Design review of the part built by this model. Coordinates are the model's own, in mm. Face numbers are marked on the shaded views. A direction names the side the tool comes from. Coordinates: 2 decimals unless noted, no trailing zeros. Loops run counter-clockwise (first coordinate to the right, second up) from the corner with the lowest first, then second, coordinate; pieces in that order, holes last. Notation, with made-up numbers: M 53,23 L 71,23 A18 ccw 71,40 Z; hole C 17.5,2.5 d2. An arc over 180 degrees is marked long. Answer as a JSON object with one key per item and string values. Group by question number.
1. Machinability: for the marked faces 1 and 2, which of the approach directions +Z, -Z, +X, -X, +Y, -Y give a long, thin tool a straight path to every point of the face, cutting with its end or side? Answer none if there is none.
2. Consider section C-C (x = 14). State the section outline as (y, z) points, then the cut area to 3 significant figures.
3. Consider section A-A (x = 0). State the section outline as (y, z) points, then the cut area to 3 significant figures.
4. To check wall thickness, follow probe 1 along Y at (x, z) = (0, 0.8); probe 2 along Y at (x, z) = (0, 3.5); probe 3 along Z at (x, y) = (4, -15). State the ranges of each line that lie inside material, in increasing order.
5. Insertion check: pin 1 (1 mm diameter, centred on x = 12, z = 1.5, fed in from +Y); pin 2 (4 mm diameter, centred on x = 14, y = 0, fed in from +Z); pin 3 (4 mm diameter, centred on y = -7, z = 1, fed in from +X). Each pin has a flat end and moves straight along its axis. Give the tip position at first contact, or say it passes through.
6. Consider section D-D (z = 1). State the section outline as (x, y) points, then the cut area to 3 significant figures.
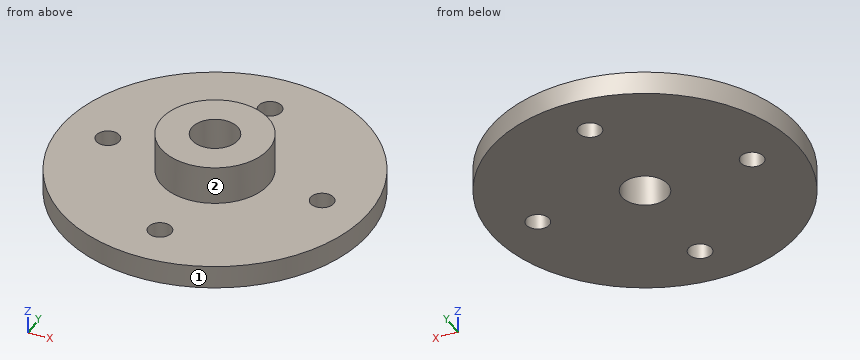
Autodesk Inventor part; units mm, degrees
ref_plane "YZ Plane" through (0, 0, 0) normal (1, 0, 0) x (0, 1, 0)
ref_plane "XZ Plane" through (0, 0, 0) normal (0, 1, 0) x (-1, 0, 0)
ref_plane "XY Plane" through (0, 0, 0) normal (0, 0, 1) x (1, 0, 0)
sketch "スケッチ1" plane through (0, 0, 0) normal (0, 0, 1) x (1, 0, 0)
  circle A0 centre (0, 0) radius 20
  dimension "d0" = 40
extrude "押し出し1" add sketch "スケッチ1" along normal blind 3
sketch "スケッチ2" plane through (0, 0, 3) normal (0, 0, 1) x (1, 0, 0)
  circle A0 centre (0, 0) radius 7
  dimension "d3" = 14
extrude "押し出し2" add sketch "スケッチ2" along normal blind 5
sketch "スケッチ3" plane through (0, 0, 8) normal (0, 0, 1) x (1, 0, 0)
  circle A0 centre (0, 0) radius 3
  dimension "d6" = 6
extrude "押し出し3" cut sketch "スケッチ3" against normal through all
sketch "スケッチ4" plane through (0, 0, 0) normal (0, 0, -1) x (-1, 0, 0)
  point P0 (0, 0)
  point P1 (0, 14)
  point P2 (0, -14)
  point P3 (14, 0)
  point P4 (-14, 0)
  dimension "d9" = 28
  dimension "d10" = 28
  dimension "d11" = 14
  dimension "d12" = 14
hole "穴1" at (0, 14, 0) at (0, -14, 0) at (-14, 0, 0) at (14, 0, 0) direction (0, 0, 1) diameter 3 end through all
sketch "スケッチ5" plane through (0, 0, 8) normal (0, 0, 1) x (1, 0, 0)
  point P0 (0, 0)
sketch "スケッチ6" plane through (0, 0, 0) normal (1, 0, 0) x (0, 1, 0)
  point P0 (0, 0)
properties part number "RD010_ギアDS0.5-80" material "PVC、無可塑"
Findings below:
{
 "1": {"face 1": "+Z, -Z", "face 2": "+Z"},
 "2": {"outline": "M -14.28,0 L -1.5,0 L -1.5,3 L -14.28,3 Z; M 1.5,0 L 14.28,0 L 14.28,3 L 1.5,3 Z", "area": "76.7 mm^2"},
 "3": {"outline": "M -20,0 L -15.5,0 L -15.5,3 L -20,3 Z; M -12.5,0 L -3,0 L -3,8 L -7,8 L -7,3 L -12.5,3 Z; M 3,0 L 12.5,0 L 12.5,3 L 7,3 L 7,8 L 3,8 Z; M 15.5,0 L 20,0 L 20,3 L 15.5,3 Z", "area": "124 mm^2"},
 "4": {"probe 1": "y = -20 to -15.5, -12.5 to -3, 3 to 12.5, 15.5 to 20", "probe 2": "y = -7 to -3, 3 to 7", "probe 3": "z = 0 to 3"},
 "5": {"pin 1": "stops at y = 16.36", "pin 2": "stops at z = 3", "pin 3": "stops at x = 19.36"},
 "6": {"outline": "C 0,0 d40; hole C -14,0 d3; hole C 0,0 d6; hole C 0,-14 d3; hole C 0,14 d3; hole C 14,0 d3", "area": "1,200 mm^2"}
}
